Source: CAD feature listing. Evaluate the final solid. Frame: model axes, mm. A direction names the side the tool comes from. Coordinates: 2 decimals unless noted, no trailing zeros. Write each loop counter-clockwise with the first axis right and the second up, starting at its lowest first coordinate (ties: lowest second). Pieces come first, ordered by that corner, then holes. Notation, with made-up numbers: M 31.5,74.25 L 55.5,74.25 A30 ccw 55.5,110.25 Z; hole C 21,18 d1. An arc over 180 degrees is marked long. Write item = value, one per line. Start each with the question number.
1. Pin query (flat end, axial travel): pin 1 Ø1.8 at (x, y) = (49, 10) entering from +Z; pin 2 Ø3 at (x, y) = (55.5, 17) entering from -Z; pin 3 Ø5 at (y, z) = (50, 5) entering from +X; pin 4 Ø8 at (x, y) = (30, 50) entering from +Z. Return the tip coordinate at first contact, or that it passes through.
2. Line query: line 1 along Y through (x, z) = (30, 12.35); line 2 along Y through (x, z) = (4.5, 8.25). Output: solid intervals per line, ascending.
3. Section query B-B (x = 22). Output: boundary loops of the cut face in (y, z).
4. Pull-direction query (Y, two-part tool) for faces 1 (the face through (30, 8, 11.5)), 2 (the face through (20, 79, 6)), 3 (the face through (27.6, 68.2, 13.3)); classes: pulls with the +Y half, pulls with the -Y half, needs draft (parallel to the pull), parting line crosses it, or undercut.
5. Access query for faces 4 (the face through (47.79, 52.03, 13.27)), 5 (the face through (31.57, 29.35, 10.27)), 6 (the face through (72, 50, 9)), 7 (the face through (12, 70, 9)), 8 (the face through (32, 70, 9)). Directions: +Z, -Z, +X, -X, +Y, -Y. A direction counts if a zero-diameter tool reaches every point of the face in a straight line with its end or side. Return the directions, or none.
6. Section query D-D (x = 30). Give the number of separate pieces and of enclosed holes in the cut face, then the cut area to 3 significant figures.
7. Section query A-A (z = 7.5). Output: boundary loops of the cut face in (x, y), then the cut area to 3 significant figures.
```python
from build123d import *

# Parameters (mm, degrees)
SKETCH_W        = 80
SKETCH_H        = 80
PAD_DEPTH       = 15
POCKET_DEPTH    = 12
SKETCH006_R     = 5
PAD001_DEPTH    = 3
SKETCH004_R     = 1.7
POCKET001_DEPTH = 10
SKETCH009_R     = 3
POCKET002_DEPTH = 3.5
FILLET_R        = 2
FILLET001_R     = 1.5


with BuildPart() as part:
    # Sketch → Pad (new body)
    with BuildSketch(Plane.XY):
        with Locations((40, 40)):
            Rectangle(SKETCH_W, SKETCH_H)
    extrude(amount=PAD_DEPTH)

    # Sketch003 (on Face5 of Pad) → Pocket (cut)
    with BuildSketch(Plane(origin=(0, 0, 0), x_dir=(1, 0, 0), z_dir=(0, 0, -1))):
        Polygon((3, -3), (77, -3), (77, -20), (80, -20), (80, -60), (77, -60), (77, -77), (60, -77), (60, -80), (20, -80), (20, -77), (3, -77), align=None)
    extrude(amount=-POCKET_DEPTH, mode=Mode.SUBTRACT)

    # Sketch006 (on Face4 of Pocket) → Pad001 (join)
    with BuildSketch(Plane(origin=(0, 0, 12), x_dir=(1, 0, 0), z_dir=(0, 0, -1))):
        with Locations((10, -10)):
            Circle(SKETCH006_R)
        with Locations((30, -10)):
            Circle(SKETCH006_R)
        with Locations((50, -10)):
            Circle(SKETCH006_R)
        with Locations((70, -10)):
            Circle(SKETCH006_R)
        with Locations((10, -30)):
            Circle(SKETCH006_R)
        with Locations((30, -30)):
            Circle(SKETCH006_R)
        with Locations((50, -30)):
            Circle(SKETCH006_R)
        with Locations((70, -30)):
            Circle(SKETCH006_R)
        with Locations((10, -50)):
            Circle(SKETCH006_R)
        with Locations((30, -50)):
            Circle(SKETCH006_R)
        with Locations((50, -50)):
            Circle(SKETCH006_R)
        with Locations((70, -50)):
            Circle(SKETCH006_R)
        with Locations((10, -70)):
            Circle(SKETCH006_R)
        with Locations((30, -70)):
            Circle(SKETCH006_R)
        with Locations((50, -70)):
            Circle(SKETCH006_R)
        with Locations((70, -70)):
            Circle(SKETCH006_R)
    extrude(amount=PAD001_DEPTH)

    # Sketch004 (on Face8 of Pad001) → Pocket001 (cut)
    with BuildSketch(Plane.XY.offset(15)):
        with Locations((10, 10)):
            Circle(SKETCH004_R)
        with Locations((10, 30)):
            Circle(SKETCH004_R)
        with Locations((10, 50)):
            Circle(SKETCH004_R)
        with Locations((10, 70)):
            Circle(SKETCH004_R)
        with Locations((30, 10)):
            Circle(SKETCH004_R)
        with Locations((30, 30)):
            Circle(SKETCH004_R)
        with Locations((30, 50)):
            Circle(SKETCH004_R)
        with Locations((30, 70)):
            Circle(SKETCH004_R)
        with Locations((50, 10)):
            Circle(SKETCH004_R)
        with Locations((50, 30)):
            Circle(SKETCH004_R)
        with Locations((50, 50)):
            Circle(SKETCH004_R)
        with Locations((50, 70)):
            Circle(SKETCH004_R)
        with Locations((70, 10)):
            Circle(SKETCH004_R)
        with Locations((70, 30)):
            Circle(SKETCH004_R)
        with Locations((70, 50)):
            Circle(SKETCH004_R)
        with Locations((70, 70)):
            Circle(SKETCH004_R)
    extrude(amount=-POCKET001_DEPTH, mode=Mode.SUBTRACT)

    # Sketch009 (on Face8 of Pocket001) → Pocket002 (cut)
    with BuildSketch(Plane.XY.offset(15)):
        with Locations((10, 10)):
            Circle(SKETCH009_R)
        with Locations((10, 30)):
            Circle(SKETCH009_R)
        with Locations((10, 50)):
            Circle(SKETCH009_R)
        with Locations((10, 70)):
            Circle(SKETCH009_R)
        with Locations((30, 10)):
            Circle(SKETCH009_R)
        with Locations((30, 30)):
            Circle(SKETCH009_R)
        with Locations((30, 50)):
            Circle(SKETCH009_R)
        with Locations((30, 70)):
            Circle(SKETCH009_R)
        with Locations((50, 10)):
            Circle(SKETCH009_R)
        with Locations((50, 30)):
            Circle(SKETCH009_R)
        with Locations((50, 50)):
            Circle(SKETCH009_R)
        with Locations((50, 70)):
            Circle(SKETCH009_R)
        with Locations((70, 10)):
            Circle(SKETCH009_R)
        with Locations((70, 30)):
            Circle(SKETCH009_R)
        with Locations((70, 50)):
            Circle(SKETCH009_R)
        with Locations((70, 70)):
            Circle(SKETCH009_R)
    extrude(amount=-POCKET002_DEPTH, mode=Mode.SUBTRACT)

    # Fillet
    fillet_edges = [part.edges().sort_by_distance(p)[0] for p in [
        (40, 0, 15),
        (0, 0, 7.5),
        (0, 40, 15),
    ]]
    fillet(fillet_edges, radius=FILLET_R)

    # Fillet001
    fillet001_edges = [part.edges().sort_by_distance(p)[0] for p in [
        (68.5, 77, 12),
        (77, 68.5, 12),
        (77, 11.5, 12),
        (40, 3, 12),
        (3, 40, 12),
        (11.5, 77, 12),
    ]]
    fillet(fillet001_edges, radius=FILLET001_R)


solid = part.part
```
Results are:
q1.pin_1 = 11.5
q1.pin_2 = 12
q1.pin_3 = 3
q1.pin_4 = 15
q2.line_1 = 0 to 7, 13 to 27, 33 to 47, 53 to 67, 73 to 80
q2.line_2 = 0 to 3, 77 to 80
q3.outline = M 0,0 L 3,0 L 3,10.5 A1.5 cw 4.5,12 L 80,12 L 80,15 L 2,15 A2 ccw 0,13 Z
q4.face_1 = undercut
q4.face_2 = needs draft
q4.face_3 = undercut
q5.face_4 = +Z
q5.face_5 = +Z, -Z
q5.face_6 = -Z, +X
q5.face_7 = -Z
q5.face_8 = -Z, +Y
q6.separate_pieces = 5
q6.enclosed_holes = 0
q6.area = 278 mm^2
q7.outline = M 0,2 A2 ccw 2,0 L 80,0 L 80,20 L 77,20 L 77,3 L 3,3 L 3,77 L 20,77 L 20,80 L 0,80 Z; M 60,77 L 77,77 L 77,60 L 80,60 L 80,80 L 60,80 Z
q7.area = 683 mm^2
